Source: three-view drawing plus pictorial views. Frame: mm from the lowest corner of the part. A direction names the side the tool comes from. Round coordinates to 2 decimals unless told otherwise and drop trailing zeros. Write each loop counter-clockwise with the first axis right and the second up, starting at its lowest first coordinate (ties: lowest second). Pieces come first, ordered by that corner, then holes.
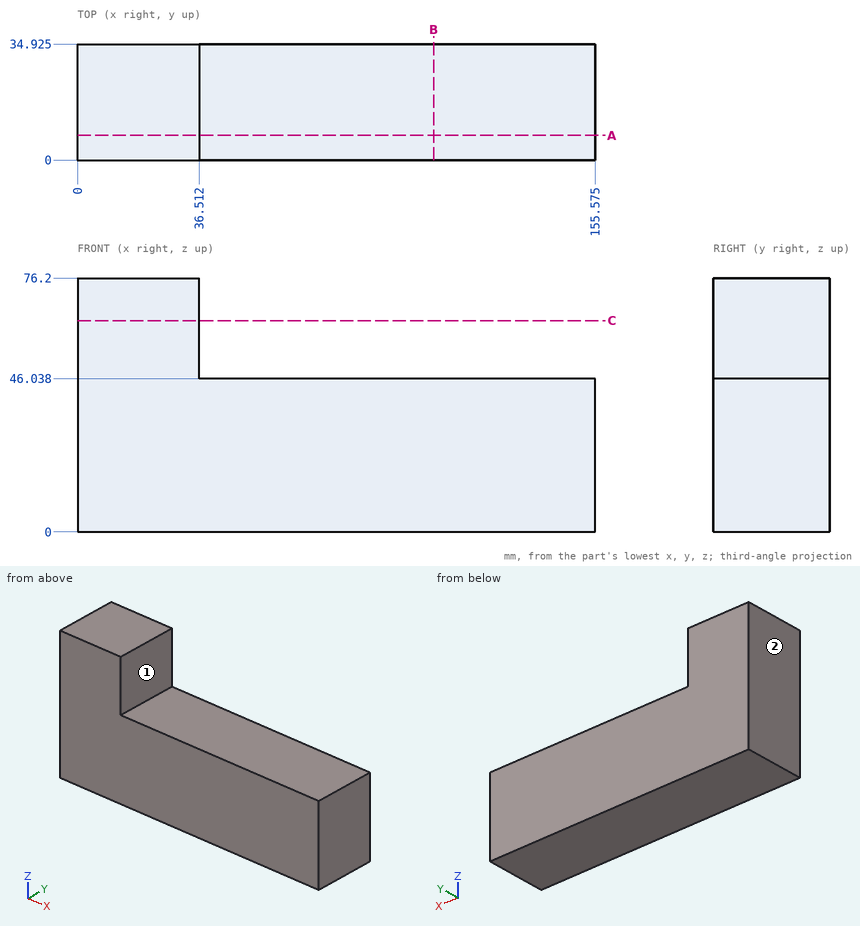
1) Section C-C on z = 63.5. Output: boundary loops of the cut face in (x, y) (1 decimal), plus the area to 3 significant figures.
2) Section A-A on y = 7.5. Output: boundary loops of the cut face in (x, z) (1 decimal).
3) Section B-B on x = 107. Output: boundary loops of the cut face in (y, z) (1 decimal).
4) Line query: probe 1 along Z at (x, y) = (135.5, 17); probe 2 along X at (y, z) = (7.5, 47.5). Output: solid intervals per line, ascending.
5) First-contact query: P1, Ø9, axis at y = 23.5, z = 55.5, coming from the +X side. Flat tip, straight axial feed; report the tip coordinate or a pass-through.
6) Reachability of the marked faces 1 and 2 from +Z, -Z, +X, -X, +Y, -Y: full face, straight path, thin tool, end or side. Return the list, or none.
Filled in:
1. outline: (0, 0) - (36.5, 0) - (36.5, 34.9) - (0, 34.9) - close
1. area: 1,280 mm2
2. outline: (0, 0) - (155.6, 0) - (155.6, 46) - (36.5, 46) - (36.5, 76.2) - (0, 76.2) - close
3. outline: (0, 0) - (34.9, 0) - (34.9, 46) - (0, 46) - close
4. probe 1: z = 0 to 46.04
4. probe 2: x = 0 to 36.51
5. P1: stops at x = 36.51
6. face 1: +Z, +X, +Y, -Y
6. face 2: +Z, -Z, -X, +Y, -Y
